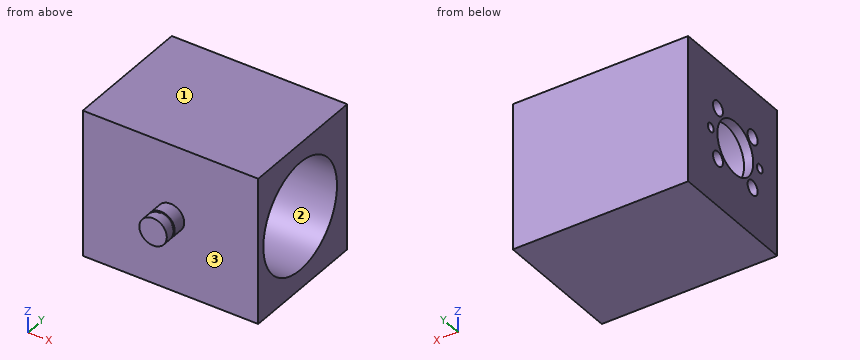
```python
from build123d import *

# Parameters (mm, degrees)
SKETCH1_W              = 60.96
SKETCH1_H              = 50.8
BOSS_EXTRUDE1_DEPTH    = 40.64
SKETCH3_W              = 60.96
SKETCH3_H              = 50.8
BOSS_EXTRUDE2_DEPTH    = 1.5875
SKETCH2_R              = 18.8
CUT_EXTRUDE1_DEPTH     = 57.785
SKETCH4_W              = 60.96
SKETCH4_H              = 50.8
BOSS_EXTRUDE3_DEPTH    = 3.175
SKETCH6_R              = 9.144
CUT_EXTRUDE2_DEPTH     = 3.175
SKETCH7_R              = 1.5
CUT_EXTRUDE3_DEPTH     = 3.175
SKETCH8_R              = 4.7625
BOSS_EXTRUDE4_DEPTH    = 8.89
CUT_EXTRUDE4_START     = -7.1501
CUT_EXTRUDE4_OUTLINE_R = 4.7625
CUT_EXTRUDE4_DEPTH     = 0.7366
SKETCH9_R              = 4.4704
BOSS_EXTRUDE5_DEPTH    = 0.7366
SKETCH13_R             = 2.54
CUT_EXTRUDE6_DEPTH     = 3.175


# Read off the part's stored shape, not the designer's step: Cut-Extrude4
with BuildPart() as part:
    # Sketch1 → Boss-Extrude1 (new body)
    with BuildSketch(Plane(origin=(0, 0, 0), x_dir=(1, 0, 0), z_dir=(0, 1, 0))):
        Rectangle(SKETCH1_W, SKETCH1_H)
    extrude(amount=BOSS_EXTRUDE1_DEPTH)

    # Sketch3 → Boss-Extrude2 (add)
    with BuildSketch(Plane(origin=(0, 0, 0), x_dir=(-1, 0, 0), z_dir=(0, -1, 0))):
        Rectangle(SKETCH3_W, SKETCH3_H)
    extrude(amount=BOSS_EXTRUDE2_DEPTH)

    # Sketch2 → Cut-Extrude1 (cut)
    with BuildSketch(Plane(origin=(30.48, 0, 0), x_dir=(0, 0, -1), z_dir=(1, 0, 0))):
        with Locations((0, 19.812)):
            Circle(SKETCH2_R)
    extrude(amount=-CUT_EXTRUDE1_DEPTH, mode=Mode.SUBTRACT)

    # Sketch4 → Boss-Extrude3 (add)
    with BuildSketch(Plane(origin=(0, 40.64, 0), x_dir=(1, 0, 0), z_dir=(0, 1, 0))):
        Rectangle(SKETCH4_W, SKETCH4_H)
    extrude(amount=BOSS_EXTRUDE3_DEPTH)

    # Sketch6 → Cut-Extrude2 (cut)
    with BuildSketch(Plane.ZY.offset(30.48)):
        with Locations((0, 19.812)):
            Circle(SKETCH6_R)
    extrude(amount=-CUT_EXTRUDE2_DEPTH, mode=Mode.SUBTRACT)

    # Sketch7 → Cut-Extrude3 (cut)
    with BuildSketch(Plane.ZY.offset(30.48)):
        with Locations((0, 32.312000019)):
            Circle(SKETCH7_R)
        with Locations((0, 7.311999981)):
            Circle(SKETCH7_R)
    extrude(amount=-CUT_EXTRUDE3_DEPTH, mode=Mode.SUBTRACT)

    # Sketch8 → Boss-Extrude4 (add)
    with BuildSketch(Plane.XZ.offset(1.5875)):
        with Locations(Location((0, 0, 0), (0, 0, 90))):
            Circle(SKETCH8_R)
    extrude(amount=BOSS_EXTRUDE4_DEPTH)

    # Cut-Extrude4 outline → Cut-Extrude4 (cut)
    with BuildSketch(Plane(origin=(0, 0, 0), x_dir=(1, 0, 0), z_dir=(0, 1, 0)).offset(CUT_EXTRUDE4_START)):
        Circle(CUT_EXTRUDE4_OUTLINE_R)
    extrude(amount=CUT_EXTRUDE4_DEPTH, mode=Mode.SUBTRACT)

    # Sketch9 → Boss-Extrude5 (add)
    with BuildSketch(Plane(origin=(0, -6.4135, 0), x_dir=(-1, 0, 0), z_dir=(0, -1, 0))):
        with Locations(Location((0, 0, 0), (0, 0, 90))):
            Circle(SKETCH9_R)
    extrude(amount=BOSS_EXTRUDE5_DEPTH)

    # Sketch13 → Cut-Extrude6 (cut)
    with BuildSketch(Plane.ZY.offset(30.48)):
        with Locations((8.838834778, 28.650834778)):
            Circle(SKETCH13_R)
        with Locations((-8.838834778, 28.650834778)):
            Circle(SKETCH13_R)
        with Locations((-8.838834778, 10.973165222)):
            Circle(SKETCH13_R)
        with Locations((8.838834778, 10.973165222)):
            Circle(SKETCH13_R)
    extrude(amount=-CUT_EXTRUDE6_DEPTH, mode=Mode.SUBTRACT)


solid = part.part
```
Check sheet for the modelled part. Datum: model origin and axes. Units: mm. Face numbers are marked on the shaded views. Coordinates: 2 decimals unless noted, no trailing zeros. Order: outer loops, then holes, each group sorted by start corner. A loop starts at its lowest first (then second) coordinate and runs counter-clockwise, first axis right, second up. Notation, with made-up numbers: (30, 28) -> (39, 28) arc R25 cw to (39, 59) -> close; hole circle Ø7 at (-22, 65). An arc over 180 degrees is marked (long way). Write each question's results on one line, items separated by ' | '. Start each with the question number.
1) Section check A-A (z = 0). Count the separate pieces of the cut face and the enclosed holes in it, and give its area (3 significant figures).
2) Material ranges on line 1 along Y through (x, z) = (-28, 0) (1 decimal); line 2 along Y through (x, z) = (0.5, 0) (1 decimal); line 3 along Z through (x, y) = (0, 20.5), recorded low to high.
3) Section check C-C (y = 15). Enter the section's corners in (x, z) (3 decimals), and give its area (3 significant figures).
4) Section check D-D (z = 17.5). Enter the section's corners in (x, y) (1 decimal), and give its area (3 significant figures).
5) Depth check by flat-ended pin: pin 1 (4.5 mm diameter, centred on y = 10.97, z = -8.84, fed in from -X); pin 2 (15 mm diameter, centred on x = 12.5, z = 10.5, fed in from -Y); pin 3 (8 mm diameter, centred on y = 10.97, z = 8.84, fed in from +X) (3 decimals). Enter the tip coordinate at first touch or a pass-through.
6) Draft check along Z on the marked faces 1, 2 and 3. Enter one of: pulls with the +Z half, pulls with the -Z half, needs draft (parallel to the pull), parting line crosses it, or undercut.
Checked values:
1) separate pieces: 4 | enclosed holes: 0 | area: 602 mm²
2) line 1: -1.6 to 5.8, 8.8 to 10.7, 29 to 30.8, 33.8 to 43.8 | line 2: -10.5 to 1, 38.6 to 43.8 | line 3: -25.4 to -18.79, 18.79 to 25.4
3) outline: (-30.48, -25.4) -> (30.48, -25.4) -> (30.48, -18.174) -> (-27.305, -18.174) -> (-27.305, -7.775) -> (-30.48, -7.775) -> close; (-30.48, 7.775) -> (-27.305, 7.775) -> (-27.305, 18.174) -> (30.48, 18.174) -> (30.48, 25.4) -> (-30.48, 25.4) -> close | area: 947 mm²
4) outline: (-30.5, -1.6) -> (30.5, -1.6) -> (30.5, 12.9) -> (-27.3, 12.9) -> (-27.3, 26.7) -> (30.5, 26.7) -> (30.5, 43.8) -> (-30.5, 43.8) -> close | area: 1,970 mm²
5) pin 1: through | pin 2: y = -1.59 | pin 3: x = -27.305
6) face 1: pulls with the +Z half | face 2: undercut | face 3: needs draft
